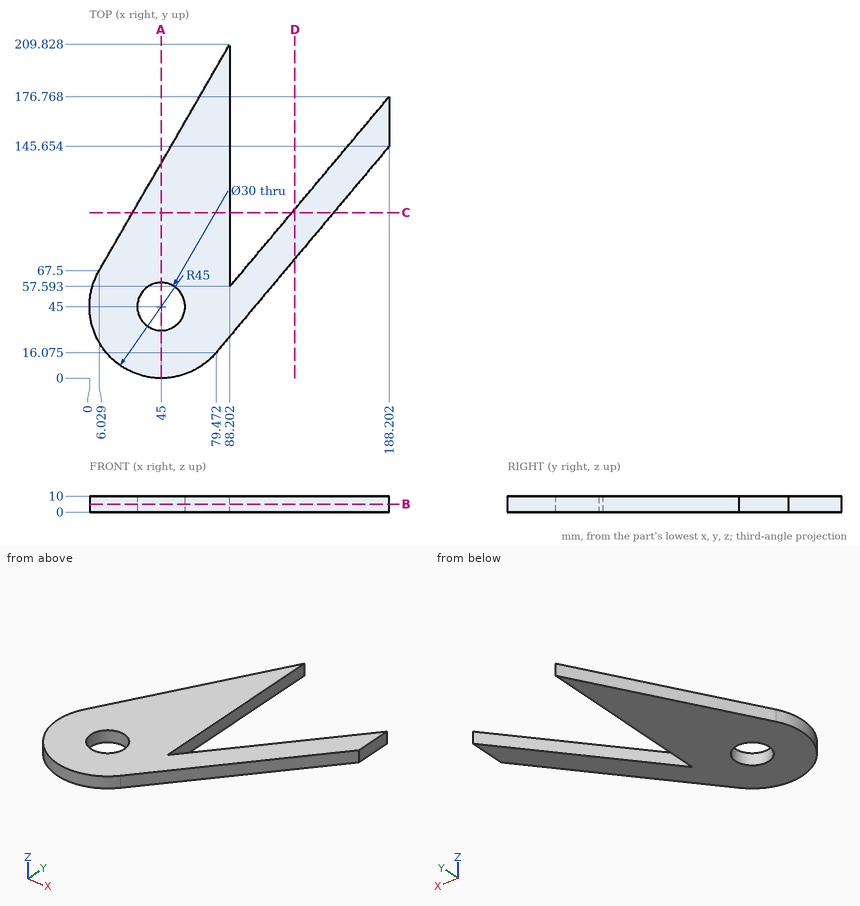
For this review, use the dimensioned drawing (mm, ordinates from the lowest corner) and the shaded views. Coordinates: 2 decimals unless noted, no trailing zeros. Loops run counter-clockwise (first coordinate to the right, second up) from the corner with the lowest first, then second, coordinate; pieces in that order, holes last. Notation, with made-up numbers: (42.25, 13) - (93.25, 13) arc R15 cw to (93.25, 29) - close; hole circle Ø10 at (-32, -2). An arc over 180 degrees is marked (long way). Use one line per item in the form item = value. Start each with the question number.
1) Take a section at A-A (x = 45). State the section outline as (y, z) points, plus the area to 3 significant figures.
2) Take a section at C-C (y = 104). State the section outline as (x, z) points, plus the area to 3 significant figures.
3) Take a section at B-B (z = 5). State the section outline as (x, y) points (1 decimal), plus the area to 3 significant figures.
4) For pin 1 (3 mm diameter, centred on y = 118, z = 2, fed in from -X); pin 2 (2 mm diameter, centred on x = 166.5, z = 3, fed in from +Y) (1 decimal); pin 3 (1.5 mm diameter, centred on x = 43.5, z = 6.5, fed in from +Y), all flat-tipped, find the tip position at first contact; note any pin that passes through.
5) Take a section at D-D (x = 129). State the section outline as (y, z) points (1 decimal), plus the area to 3 significant figures.
6) To check wall thickness, follow probe 1 along Y at (x, z) = (45, 4.25); probe 2 along X at (y, z) = (175, 2.5) (1 decimal); probe 3 along X at (y, z) = (144, 6.25) (1 decimal). State the ranges of each line that lie inside material, in increasing order. Write a range as from..to.
From the geometry:
q1.outline = (0, 0) - (30, 0) - (30, 10) - (0, 10) - close; (60, 0) - (135, 0) - (135, 10) - (60, 10) - close
q1.area = 1,050 mm2
q2.outline = (27.1, 0) - (88.2, 0) - (88.2, 10) - (27.1, 10) - close; (127.14, 0) - (153.25, 0) - (153.25, 10) - (127.14, 10) - close
q2.area = 872 mm2
q3.outline = (6, 67.5) arc R45 ccw to (79.5, 16.1) - (188.2, 145.7) - (188.2, 176.8) - (88.2, 57.6) - (88.2, 209.8) - close; hole circle Ø30 at (45, 45)
q3.area = 13,400 mm2
q4.pin_1 = 34.32
q4.pin_2 = 152.1
q4.pin_3 = 133.7
q5.outline = (75.1, 0) - (106.2, 0) - (106.2, 10) - (75.1, 10) - close
q5.area = 311 mm2
q6.probe_1 = 0..30, 60..135
q6.probe_2 = 68.1..88.2, 186.7..188.2
q6.probe_3 = 50.2..88.2, 160.7..186.8
